Verification items for the finished model (mm, model axes). Face numbers are marked on the shaded views. A direction names the side the tool comes from. Coordinates: 2 decimals unless noted, no trailing zeros. Loops run counter-clockwise (first coordinate to the right, second up) from the corner with the lowest first, then second, coordinate; pieces in that order, holes last. Notation, with made-up numbers: (34, -19.5) - (49, -19.5) arc R19 ccw to (49, 15.5) - close; hole circle Ø4 at (-22.75, -11.75). An arc over 180 degrees is marked (long way). One line per item, written item: value. Start each with the question number.
(1) Section check B-B (y = 3.5). Record the boundary of the cut face in (x, z), plus the area to 3 significant figures.
(2) Thickness scan on probe 1 along Z at (x, y) = (10.5, -0.5); probe 2 along Z at (x, y) = (-11, 5.5); probe 3 along X at (y, z) = (8.25, -3). Record the ranges inside material, lowest first. Write a range as [from, to].
(3) Set-up check for the marked faces 1, 2 and 3: record each of +Z, -Z, +X, -X, +Y, -Y from which the full face is reachable in a straight line by a thin tool's end or side.
(4) Section check C-C (z = 0.25). Count the separate pieces of the cut face and the enclosed holes in it, plus the area to 3 significant figures.
(5) Draft check along Z on the marked faces 4, 5, 6 and 7. Enter one of: +Z half, -Z half, draft (parallel to the pull), parting line (faces both ways), or undercut.
(6) Gauge pin test, flat ends, axial feed: P1, Ø4, axis at x = 15, y = 7, coming from the -Z side; P2, Ø4, axis at x = -20.5, z = -1.5, coming from the -Y side; P3, Ø4.5, axis at x = -17.56, z = -0.31, coming from the -Y side. Record the tip position at first contact, or that the pin passes through.
(7) Section check D-D (y = -6.25). Record the boundary of the cut face in (x, z), plus the area to 3 significant figures.
(8) Section check A-A (y = 6.75). Record the boundary of the cut face in (x, z).
```python
from build123d import *

# Parameters (mm, degrees)
EXTRUDE_1_DEPTH     = 10
EXTRUDE_1_2_DEPTH   = 10
EXTRUDE_3_DEPTH     = 11.703576761
SKETCH_5_R          = 1.7
CUT_EXTRUDE_1_DEPTH = 27.289015437
CUT_EXTRUDE_2_DEPTH = 2.4


with BuildPart() as part:
    # Sketch 1 → Extrude 1 (new body)
    with BuildSketch(Plane(origin=(0, 0, 0), x_dir=(1, 0, 0), z_dir=(0, 1, 0))):
        with BuildLine():
            Line((10.893392623, -6.049715663), (18.526323659, -6.186490707))
            ThreePointArc((18.526323659, -6.186490707), (23.511587835, -0.423094228), (18.736007239, 5.515207537))
            Line((18.736007239, 5.515207537), (11.103076203, 5.651982581))
            Line((11.103076203, 5.651982581), (10.893392623, -6.049715663))
        make_face()
    extrude(amount=EXTRUDE_1_DEPTH)



with BuildPart() as body_2:
    # Sketch 1 → Extrude 1 2 (new body)
    with BuildSketch(Plane(origin=(0, 0, 0), x_dir=(1, 0, 0), z_dir=(0, 1, 0))):
        with BuildLine():
            Line((-10.893392623, 6.046138902), (-18.526323659, 6.182913947))
            ThreePointArc((-18.526323659, 6.182913947), (-23.511587835, 0.419517467), (-18.736007239, -5.518784297))
            Line((-18.736007239, -5.518784297), (-11.103076203, -5.655559342))
            Line((-11.103076203, -5.655559342), (-10.893392623, 6.046138902))
        make_face()
    extrude(amount=EXTRUDE_1_2_DEPTH)


with BuildPart() as part_1:
    add(part.part)

    add(body_2.part)  # Extrude 3 merges body 2
    # Sketch 3 → Extrude 3 (add)
    with BuildSketch(Plane(origin=(-0.104873826, 0, 5.852636928), x_dir=(0.9998394920722602, 0, 0.017916196378829744), z_dir=(-0.017916196378829744, 0, 0.9998394920722602))):
        with BuildLine():
            Line((-11, 10), (-18.634156379, 10))
            ThreePointArc((-18.634156379, 10), (0, -8.634156379), (18.634156379, 10))
            Line((18.634156379, 10), (11, 10))
            ThreePointArc((11, 10), (0, -1), (-11, 10))
        make_face()
    extrude(amount=-EXTRUDE_3_DEPTH)

    # Sketch 5 → Cut-Extrude 1 (cut, through all)
    with BuildSketch(Plane.XZ):
        with Locations(Location((-17.564258534, -0.312946842, 0), (0, 0, 270))):
            Circle(SKETCH_5_R)
        with Locations(Location((17.564258534, -0.312946842, 0), (0, 0, 90))):
            Circle(SKETCH_5_R)
    extrude(amount=-CUT_EXTRUDE_1_DEPTH, mode=Mode.SUBTRACT)

    # Sketch 6 → Cut-Extrude 2 (cut, symmetric)
    with BuildSketch(Plane.XZ):
        Polygon((20.314258534, -1.900660082), (17.564258534, -3.488373323), (14.814258534, -1.900660082), (14.814258534, 1.274766398), (17.564258534, 2.862479638), (20.314258534, 1.274766398), align=None)
        Polygon((-17.564258534, -3.488373323), (-14.814258534, -1.900660082), (-14.814258534, 1.274766398), (-17.564258534, 2.862479638), (-20.314258534, 1.274766398), (-20.314258534, -1.900660082), align=None)
    extrude(amount=CUT_EXTRUDE_2_DEPTH, both=True, mode=Mode.SUBTRACT)


solid = part_1.part
```
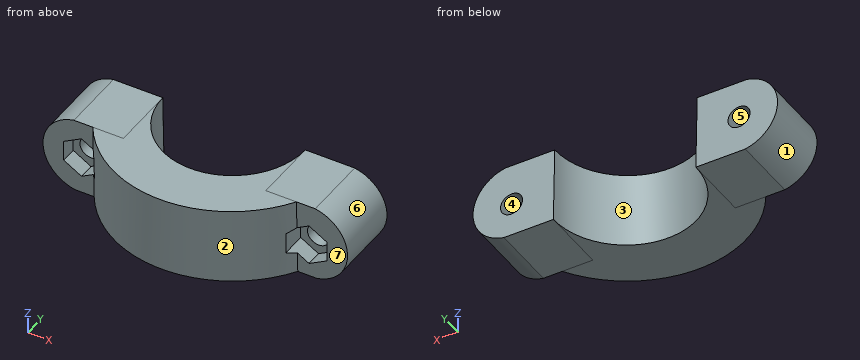
Responses:
1. outline: (-18.74, 5.52) arc R5.95 ccw to (-18.53, -6.18) - (-8.77, -6.01) - (-8.98, 5.69) - close; (8.77, 6.01) - (8.98, -5.69) - (18.74, -5.52) arc R5.95 ccw to (18.53, 6.19) - close; hole circle Ø3.4 at (-17.56, -0.31); hole circle Ø3.4 at (17.56, -0.31)
1. area: 296 mm²
2. probe 1: z = [-5.66, 6.04]
2. probe 2: z = [-6.05, 5.66]
2. probe 3: x = [-22.87, -10.81], [10.92, 22.5]
3. face 1: -X, +Y, -Y
3. face 2: -Y
3. face 3: +Y
4. separate pieces: 3
4. enclosed holes: 0
4. area: 395 mm²
5. face 4: undercut
5. face 5: undercut
5. face 6: parting line
5. face 7: draft
6. P1: stops at z = -5.62
6. P2: stops at y = 0
6. P3: stops at y = 2.4
7. outline: (-9.22, 5.69) - (-9.01, -6.01) - (9.22, -5.69) - (9.01, 6.02) - close
7. area: 213 mm²
8. outline: (-18.74, 5.52) arc R5.95 ccw to (-18.53, -6.18) - (-10.4, -6.04) - (-10.61, 5.66) - close; (10.4, 6.04) - (10.61, -5.66) - (18.74, -5.52) arc R5.95 ccw to (18.53, 6.19) - close; hole circle Ø3.4 at (-17.56, -0.31); hole circle Ø3.4 at (17.56, -0.31)
